Source: CAD feature listing. Evaluate the final solid. Frame: model axes, mm. A direction names the side the tool comes from. Round coordinates to 2 decimals unless told otherwise and drop trailing zeros. Loops run counter-clockwise (first coordinate to the right, second up) from the corner with the lowest first, then second, coordinate; pieces in that order, holes last. Notation, with made-up numbers: (-17, 45) - (38, 45) arc R12 cw to (38, 67) - close; hole circle Ø5 at (36.25, -21.5). An arc over 180 degrees is marked (long way). One line per question, with ' | ' between items.
from build123d import *

# Parameters (mm, degrees)
F1_DEPTH = 40
F3_DEPTH = 20
F4_R     = 19.99999
F5_R     = 10
F6_DEPTH = 25


# Not quite as in the source:
# - a fillet or chamfer is up to 0.001 mm smaller than in the source, because OpenCascade refuses the exact size


with BuildPart() as f1:
    # F0 (on Top) → F1 (new body)
    with BuildSketch(Plane.XY):
        Polygon((10, 40), (10, 0), (30, 0), (30, 40), (40, 40), (40, 80), (30, 80), (30, 120), (10, 120), (10, 80), (0, 80), (0, 40), align=None)
    extrude(amount=F1_DEPTH)

    # F2 (on face) → F3 (cut)
    with BuildSketch(Plane.YZ.offset(30)):
        with BuildLine():
            ThreePointArc((20, 0), (5.8578643763, 5.8578643763), (0, 20))
            Line((0, 20), (0, 0))
            Line((0, 0), (20, 0))
        make_face()
        with BuildLine():
            ThreePointArc((0, 20), (5.8578643763, 34.1421356237), (20, 40))
            Line((20, 40), (0, 40))
            Line((0, 40), (0, 20))
        make_face()
    extrude(amount=-F3_DEPTH, mode=Mode.SUBTRACT)

    # F4 (radius 20 in the source; OpenCascade refuses exactly that, so slightly less here)
    f4_edges = [f1.edges().sort_by_distance(p)[0] for p in [
        (20, 120, 0),
        (20, 120, 40),
    ]]
    fillet(f4_edges, radius=F4_R)

    # F5 (on face) → F6 (cut)
    with BuildSketch(Plane.YZ.offset(30)):
        with Locations((100, 20)):
            Circle(F5_R)
        with Locations((20, 20)):
            Circle(F5_R)
    extrude(amount=-F6_DEPTH, mode=Mode.SUBTRACT)


solid = f1.part
1. Section query C-C, the plane x = 6. Return loops of the section in (y, z).
Worked out:
outline: (40, 0) - (80, 0) - (80, 40) - (40, 40) - close
2. Section query A-A, the plane y = 98. Return loops of the section in (x, z).
Worked out:
outline: (10, 0) - (30, 0) - (30, 10.2) - (10, 10.2) - close; (10, 29.8) - (30, 29.8) - (30, 40) - (10, 40) - close
3. Section query B-B, the plane x = 28.5. Give the number of separate pieces and of enclosed holes in the cut face, plus the area to 3 significant figures.
Worked out:
separate pieces: 1 | enclosed holes: 2 | area: 3,830 mm2
4. Contact query for flat-ended pins moving along their axis: P1, Ø8, axis at x = 4.5, z = 33.5, coming from the -Y side; P2, Ø1, axis at x = 18, z = 18.5, coming from the +Y side (3 decimals); P3, Ø20, axis at y = 97, z = 28, coming from the -X side. Output: stop coordinate, or through.
Worked out:
P1: stops at y = 40 | P2: stops at y = 119.975 | P3: stops at x = 10
5. Section query D-D, the plane z = 4.5. Return loops of the section in (x, y), plus the area to 3 significant figures.
Worked out:
outline: (0, 40) - (10, 40) - (10, 7.36) - (30, 7.36) - (30, 40) - (40, 40) - (40, 80) - (30, 80) - (30, 112.64) - (10, 112.64) - (10, 80) - (0, 80) - close | area: 2,910 mm2
6. Mould query, pull axis Y, two halves, no side actions, for faces 1 (the cylindrical face through (19.86, 113.986, 34.297)), 2 (the cylindrical face through (20.14, 92.63, 26.76)), 3 (the flat face through (5, 40, 20)), 4 (the flat face through (40, 60, 20)). Classes: released by +Y, released by -Y, zero draft, split by the parting line, or undercut.
Worked out:
face 1: released by +Y | face 2: undercut | face 3: released by -Y | face 4: zero draft
7. Material intervals for probe 1 along Z at (x, y) = (16.75, 20); probe 2 along X at (y, z) = (39, 23); probe 3 along Y at (x, z) = (22, 24.5), sorted ascending.
Worked out:
probe 1: z = 0 to 10, 30 to 40 | probe 2: x = 10 to 30 | probe 3: y = 0.51 to 11.07, 28.93 to 91.07, 108.93 to 119.49
8. Access query for faces 5 (the flat face through (10, 29, 15)), 6 (the flat face through (35, 80, 20)), 7 (the flat face through (35, 40, 20)), 8 (the flat face through (5, 80, 20)). Directions: +Z, -Z, +X, -X, +Y, -Y. A direction counts if a zero-diameter tool reaches every point of the face in a straight line with its end or side. Return the directions, or none.
Worked out:
face 5: +Z, -Z, -X, -Y | face 6: +Z, -Z, +X, +Y | face 7: +Z, -Z, +X, -Y | face 8: +Z, -Z, -X, +Y
